Read the model definition and answer for the solid it produces. Units are mm, in the model's axes. Coordinates: 2 decimals unless noted, no trailing zeros. Order: outer loops, then holes, each group sorted by start corner. A loop starts at its lowest first (then second) coordinate and runs counter-clockwise, first axis right, second up. Notation, with made-up numbers: M 74.5,63 L 125.5,63 A12 cw 125.5,69 Z; hole C 72,51.25 d9. An arc over 180 degrees is marked long. Put each result on its own line as item: value.
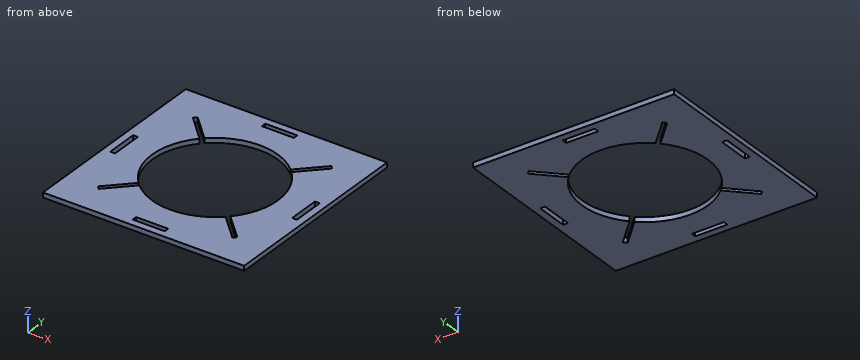
from build123d import *

# Parameters (mm, degrees)
SKETCH1_W           = 250
SKETCH1_H           = 250
BOSS_EXTRUDE1_DEPTH = 6
SKETCH2_R           = 78.2
CUT_EXTRUDE1_DEPTH  = 177.878489365
CUT_EXTRUDE2_DEPTH  = 177.878489365
CIRPATTERN1_COUNT   = 4
SKETCH4_W           = 40
SKETCH4_H           = 6
CUT_EXTRUDE3_DEPTH  = 177.878489365
CIRPATTERN2_COUNT   = 4


with BuildPart() as part:
    # Sketch1 → Boss-Extrude1 (new body)
    with BuildSketch(Plane.XY):
        Rectangle(SKETCH1_W, SKETCH1_H)
    extrude(amount=BOSS_EXTRUDE1_DEPTH)

    # Sketch2 → Cut-Extrude1 (cut, through all)
    with BuildSketch(Plane.XY.offset(6)):
        Circle(SKETCH2_R)
    extrude(amount=-CUT_EXTRUDE1_DEPTH, mode=Mode.SUBTRACT)

    # Sketch3 → Cut-Extrude2 (cut, through all)
    with BuildSketch(Plane.XY.offset(6)):
        with BuildLine():
            Line((-57.035252874, 53.499718968), (-86.620580695, 83.085046789))
            Line((-86.620580695, 83.085046789), (-83.085046789, 86.620580695))
            Line((-83.085046789, 86.620580695), (-53.499718968, 57.035252874))
            ThreePointArc((-53.499718968, 57.035252874), (-55.295750289, 55.295750289), (-57.035252874, 53.499718968))
        make_face()
    cut_extrude2 = extrude(amount=-CUT_EXTRUDE2_DEPTH, mode=Mode.SUBTRACT)

    # CirPattern1: Cut-Extrude2 ×4 about axis
    cirpattern1_axis = Axis((0, 0, 0), (0, 0, 1))
    for i in range(1, CIRPATTERN1_COUNT):
        add(cut_extrude2.rotate(cirpattern1_axis, i * 360 / CIRPATTERN1_COUNT), mode=Mode.SUBTRACT)

    # Sketch4 → Cut-Extrude3 (cut, through all)
    with BuildSketch(Plane.XY.offset(6)):
        with Locations((0, 113)):
            Rectangle(SKETCH4_W, SKETCH4_H)
    cut_extrude3 = extrude(amount=-CUT_EXTRUDE3_DEPTH, mode=Mode.SUBTRACT)

    # CirPattern2: Cut-Extrude3 ×4 about axis
    cirpattern2_axis = Axis((0, 0, 0), (0, 0, 1))
    for i in range(1, CIRPATTERN2_COUNT):
        add(cut_extrude3.rotate(cirpattern2_axis, i * 360 / CIRPATTERN2_COUNT), mode=Mode.SUBTRACT)


solid = part.part
Q1. Find section D-D on z = 4.5. Give the number of separate pieces and of enclosed holes in the cut face, plus the area to 3 significant figures.
Answers below:
separate pieces: 1
enclosed holes: 5
area: 41,500 mm^2
Q2. Find section B-B on y = -1. Write down the section's boundary in (x, z), plus the area to 3 significant figures.
Answers below:
outline: M -125,0 L -116,0 L -116,6 L -125,6 Z; M -110,0 L -78.19,0 L -78.19,6 L -110,6 Z; M 78.19,0 L 110,0 L 110,6 L 78.19,6 Z; M 116,0 L 125,0 L 125,6 L 116,6 Z
area: 490 mm^2
Q3. Consider line 1 along Y through (x, z) = (-72, 0.5); line 2 along X through (y, z) = (-10, 3); line 3 along Y through (x, z) = (14, 2.75). Determine where each line is inside the solid, lowest interval first.
Answers below:
line 1: y = -125 to -75.54, -68.46 to -30.52, 30.52 to 68.46, 75.54 to 125
line 2: x = -125 to -116, -110 to -77.56, 77.56 to 110, 116 to 125
line 3: y = -125 to -116, -110 to -76.94, 76.94 to 110, 116 to 125
Q4. Find section A-A on y = -26. Write down the section's boundary in (x, z).
Answers below:
outline: M -125,0 L -73.75,0 L -73.75,6 L -125,6 Z; M 73.75,0 L 125,0 L 125,6 L 73.75,6 Z
